Part model, mm, in its own coordinate system. A direction names the side the tool comes from. Round coordinates to 2 decimals unless told otherwise and drop trailing zeros. Loops run counter-clockwise (first coordinate to the right, second up) from the corner with the lowest first, then second, coordinate; pieces in that order, holes last.
1) 3-axis set-ups, long thin cutter, end or side, ignore diameter. For faces 1 (the flat face through (-9, 0, -163)), 2 (the flat face through (-10, 3.175, -163)): which of +Z, -Z, +X, -X, +Y, -Y reach the whole face in a straight line?
2) Band-saw the part on B-B, the plane z = -43.5. Write the cut outline in (x, y) (3 decimals), then the cut area to 3 significant figures.
3) Probe line 1 (X direction, y = 9, z = -243.5) (3 decimals); line 2 (Y direction, x = -15, z = -120.5) (3 decimals). List the from-to ranges inside material, lowest first.
4) Band-saw the part on C-C, the plane z = -132.5. Write the cut outline in (x, y) (3 decimals).
5) Mould opens along X. For faces 3 (the flat face through (-3.175, 17, -163)), 4 (the flat face through (-31.75, 16, -163)), 5 (the flat face through (-15, 3, 0)) say: +X half, -X half, draft (parallel to the pull), parting line (faces both ways), or undercut.
6) Band-saw the part on A-A, the plane y = 29. Write the cut outline in (x, z) (3 decimals).
7) Band-saw the part on D-D, the plane x = -7.5. Write the cut outline in (y, z) (3 decimals), then the cut area to 3 significant figures.
8) Drop a flat-ended pin along its axis: P1, Ø1, axis at x = -22.5, y = 4, coming from the +Z side. Give the stop position or say it passes through.
Autodesk Inventor part; units mm, degrees
ref_plane "YZ Plane" through (0, 0, 0) normal (1, 0, 0) x (0, 1, 0)
ref_plane "XZ Plane" through (0, 0, 0) normal (0, 1, 0) x (-1, 0, 0)
ref_plane "XY Plane" through (0, 0, 0) normal (0, 0, 1) x (1, 0, 0)
sketch "Sketch1" plane through (0, 0, 0) normal (0, 1, 0) x (-1, 0, 0)
  line L0 (0, 0) -> (31.75, 0)
  line L1 (31.75, 0) -> (31.75, -330.2)
  line L2 (31.75, -330.2) -> (0, -330.2)
  line L3 (0, -330.2) -> (0, 0)
  dimension "d0" = 31.75
  dimension "d1" = 330.2
extrude "Extrusion1" add sketch "Sketch1" along normal blind 3.175
sketch "Sketch8" plane through (0, 3.175, 0) normal (0, 1, 0) x (1, 0, 0)
  line L0 (-31.75, 330.2) -> (-31.75, 0)
  line L1 (-31.75, 0) -> (-28.575, 0)
  line L2 (-31.75, 0) -> (0, 0)
  line L3 (0, 0) -> (-3.175, 0)
  line L4 (-3.175, 0) -> (-3.175, 330.2)
  line L5 (0, 330.2) -> (-31.75, 330.2)
  line L6 (-3.175, 330.2) -> (0, 330.2)
  line L7 (-31.75, 330.2) -> (-28.575, 330.2)
  line L8 (-28.575, 330.2) -> (-28.575, 0)
  line L9 (0, 0) -> (0, 330.2)
  dimension "d41" = 3.175
  dimension "d42" = 3.175
extrude "Extrusion7" add sketch "Sketch8" along normal blind 28.575 contours L5 L8 L1 L0 | L5 L9 L2 L4
sketch "Sketch10" plane through (0, 0, 0) normal (0, -1, 0) x (1, 0, 0)
  line L0 (0, 0) -> (-31.75, 0)
  line L1 (-3.175, -330.2) -> (-28.575, -330.2)
  line L2 (0, -330.2) -> (0, 0)
  line L3 (-31.75, 0) -> (-31.75, -330.2)
  circle A0 centre (-15.875, -162.2821) radius 4.2545
  line L4 (0, -162.2821) -> (-31.75, -162.2821)
  dimension "d60" = 8.509
extrude "Extrusion11" cut sketch "Sketch10" against normal through all contours L4 A0 | A0 L4
sketch "Sketch12" plane through (0, 0, 0) normal (1, 0, 0) x (0, 0, -1)
  line L0 (0, 0) -> (0, 31.75)
  line L1 (330.2, 3.175) -> (330.2, 31.75)
  line L2 (330.2, 31.75) -> (0, 31.75)
  line L3 (330.2, 0) -> (0, 0)
  line L4 (12.7, 19.05) -> (12.7, 12.7)
  arc A0 (53.975, 12.7) -> (53.975, 19.05) centre (53.975, 15.875) ccw
  line L5 (12.7, 19.05) -> (53.975, 19.05)
  line L6 (12.7, 12.7) -> (53.975, 12.7)
  line L7 (317.5, 19.05) -> (317.5, 12.7)
  arc A1 (276.225, 19.05) -> (276.225, 12.7) centre (276.225, 15.875) ccw
  line L8 (276.225, 19.05) -> (317.5, 19.05)
  line L9 (317.5, 12.7) -> (276.225, 12.7)
extrude "Extrusion13" cut sketch "Sketch12" against normal through all
properties part number "Teemoverthing" material "Aluminum 6061"
Reported:
1. face 1: +Z, -Z, +X, -X, -Y
1. face 2: +Z, -Z, +Y
2. outline: (-31.75, 0) - (0, 0) - (0, 12.7) - (-3.175, 12.7) - (-3.175, 3.175) - (-28.575, 3.175) - (-28.575, 12.7) - (-31.75, 12.7) - close; (-31.75, 19.05) - (-28.575, 19.05) - (-28.575, 31.75) - (-31.75, 31.75) - close; (-3.175, 19.05) - (0, 19.05) - (0, 31.75) - (-3.175, 31.75) - close
2. area: 242 mm2
3. line 1: x = -31.75 to -28.575, -3.175 to 0
3. line 2: y = 0 to 3.175
4. outline: (-31.75, 0) - (0, 0) - (0, 31.75) - (-3.175, 31.75) - (-3.175, 3.175) - (-28.575, 3.175) - (-28.575, 31.75) - (-31.75, 31.75) - close
5. face 3: undercut
5. face 4: -X half
5. face 5: draft
6. outline: (-31.75, -330.2) - (-28.575, -330.2) - (-28.575, 0) - (-31.75, 0) - close; (-3.175, -330.2) - (0, -330.2) - (0, 0) - (-3.175, 0) - close
7. outline: (0, -330.2) - (3.175, -330.2) - (3.175, 0) - (0, 0) - close
7. area: 1,050 mm2
8. P1: passes through
